from build123d import *

# Parameters (mm, degrees)
SKETCH2_R           = 2.25
BOSS_EXTRUDE1_DEPTH = 1.3
SKETCH3_W           = 4.890037446
SKETCH3_H           = 0.8
CUT_EXTRUDE1_DEPTH  = 0.8
SKETCH4_R           = 1.5
BOSS_EXTRUDE2_DEPTH = 7
SKETCH5_R           = 0.85
BOSS_EXTRUDE3_DEPTH = 3


with BuildPart() as part:
    # Sketch2 → Boss-Extrude1 (new body)
    with BuildSketch(Plane.XY):
        Circle(SKETCH2_R)
    extrude(amount=BOSS_EXTRUDE1_DEPTH)

    # Sketch3 → Cut-Extrude1 (cut)
    with BuildSketch(Plane.XY.offset(1.3)):
        Rectangle(SKETCH3_W, SKETCH3_H)
    extrude(amount=-CUT_EXTRUDE1_DEPTH, mode=Mode.SUBTRACT)

    # Sketch4 → Boss-Extrude2 (add)
    with BuildSketch(Plane(origin=(0, 0, 0), x_dir=(-1, 0, 0), z_dir=(0, 0, -1))):
        Circle(SKETCH4_R)
    extrude(amount=BOSS_EXTRUDE2_DEPTH)

    # Sketch5 → Boss-Extrude3 (add)
    with BuildSketch(Plane(origin=(0, 0, -7), x_dir=(-1, 0, 0), z_dir=(0, 0, -1))):
        with Locations(Location((0, 0, 0), (0, 0, 180))):
            Circle(SKETCH5_R)
    extrude(amount=BOSS_EXTRUDE3_DEPTH)


solid = part.part
The listing builds one solid part. Answer for the finished solid, in the listing's coordinates (mm). A direction names the side the tool comes from. Round coordinates to 2 decimals unless told otherwise and drop trailing zeros. Write each loop counter-clockwise with the first axis right and the second up, starting at its lowest first coordinate (ties: lowest second). Pieces come first, ordered by that corner, then holes. Notation, with made-up numbers: (52.5, 81) - (106.5, 81) arc R8 ccw to (106.5, 88) - close; hole circle Ø9 at (63.5, 32). An arc over 180 degrees is marked (long way). Use a Markdown table: item, result. Add a question column.
1. The part is cut by section B-B (x = 1.7). Write down the section's boundary in (y, z), and give its area (3 significant figures).
2. Consider line 1 (Z direction, x = 1.75, y = 0.65); line 2 (Z direction, x = -0.15, y = -1.4); line 3 (Y direction, x = -0.1, z = -1.5). Determine where each line is inside the solid, lowest interval first.
3. A flat-ended cylindrical pin translates along its axis: P1, Ø1.3, axis at x = -1, y = 0, coming from the -Z side. Find the tip coordinate at first contact, or state that the pin passes through.
4. A tool of negligible diameter and unlimited length cuts with its end or side. For faces 1 (the face through (-2, 0, 0)), 2 (the face through (0, 0, 0.5)), 3 (the face through (0, 0, -10)), from which of +Z, -Z, +X, -X, +Y, -Y can it reach the whole face along a straight path? Write none if from no direction.
5. The part is cut by section C-C (z = -8.75). Write down the section's boundary in (x, y), and give its area (3 significant figures).
6. The part is cut by section A-A (y = 0). Write down the section's boundary in (x, z), and give its area (4 significant figures).
7. The part is cut by section D-D (y = 1). Write down the section's boundary in (x, z).
Reported:
| question | item | result |
|---|---|---|
| 1 | outline | (-1.47, 0) - (1.47, 0) - (1.47, 1.3) - (0.4, 1.3) - (0.4, 0.5) - (-0.4, 0.5) - (-0.4, 1.3) - (-1.47, 1.3) - close |
| 1 | area | 3.19 mm^2 |
| 2 | line 1 | 0 to 1.3 |
| 2 | line 2 | -7 to 1.3 |
| 2 | line 3 | -1.5 to 1.5 |
| 3 | P1 | z = -10 |
| 4 | face 1 | -Z |
| 4 | face 2 | +Z, +X, -X |
| 4 | face 3 | -Z, +X, -X, +Y, -Y |
| 5 | outline | circle Ø1.7 at (0, 0) |
| 5 | area | 2.27 mm^2 |
| 6 | outline | (-2.25, 0) - (-1.5, 0) - (-1.5, -7) - (-0.85, -7) - (-0.85, -10) - (0.85, -10) - (0.85, -7) - (1.5, -7) - (1.5, 0) - (2.25, 0) - (2.25, 0.5) - (-2.25, 0.5) - close |
| 6 | area | 28.35 mm^2 |
| 7 | outline | (-2.02, 0) - (-1.12, 0) - (-1.12, -7) - (1.12, -7) - (1.12, 0) - (2.02, 0) - (2.02, 1.3) - (-2.02, 1.3) - close |
